```python
from build123d import *

# Parameters (mm, degrees)
SKETCH_1_W               = 31.1
SKETCH_1_H               = 31.1
SKETCH_1_W_2             = 21.1
SKETCH_1_H_2             = 21.1
EXTRUDE_1_DEPTH          = 60
SKETCH_2_R               = 1.55
CUT_EXTRUDE_1_DEPTH      = 73.445979875
CUT_EXTRUDE_2_DEPTH      = 71.444446197
CUT_EXTRUDE_2_DEPTH_BACK = 71.444446197
SKETCH_3_W               = 2.7
SKETCH_3_H               = 6
SKETCH_4_R               = 1.55
CUT_EXTRUDE_3_DEPTH      = 73.445979875
CUT_EXTRUDE_4_DEPTH      = 71.444446197
CUT_EXTRUDE_4_DEPTH_BACK = 71.444446197
SKETCH_5_W               = 3.5
SKETCH_5_H               = 6.2
FILLET_1_R               = 1.5
SKETCH_6_W               = 20.2
SKETCH_6_H               = 20.2
CUT_EXTRUDE_5_DEPTH      = 73.445979875
SKETCH_7_R               = 1.55
EXTRUDE_2_DEPTH          = 2.25
EXTRUDE_START            = 2.25
SKETCH_8_R               = 1.55
EXTRUDE_3_DEPTH          = 2.25


with BuildPart() as part:
    # 草图1 → 凸台-拉伸1 (new body)
    with BuildSketch(Plane(origin=(0, 0, 0), x_dir=(1, 0, 0), z_dir=(0, 1, 0))):
        with Locations((10.55, 10.55)):
            Rectangle(SKETCH_1_W, SKETCH_1_H)
        with Locations((10.55, 10.55)):
            Rectangle(SKETCH_1_W_2, SKETCH_1_H_2, mode=Mode.SUBTRACT)
    extrude(amount=EXTRUDE_1_DEPTH)

    # 草图2 → 切除-拉伸1 (cut, through all)
    with BuildSketch(Plane.ZY.offset(5)):
        with Locations((-23.6, 57)):
            Circle(SKETCH_2_R)
        with Locations((-23.6, 3)):
            Circle(SKETCH_2_R)
        with Locations((2.5, 3)):
            Circle(SKETCH_2_R)
        with Locations((2.5, 57)):
            Circle(SKETCH_2_R)
    extrude(amount=-CUT_EXTRUDE_1_DEPTH, mode=Mode.SUBTRACT)

    # 草图3 → 切除-拉伸2 (cut, two sides: drawn at the far end of the back side and taken through both)
    with BuildSketch(Plane.XY.offset(-21.1).offset(-CUT_EXTRUDE_2_DEPTH_BACK)):
        with Locations((6.2, 57)):
            Rectangle(SKETCH_3_W, SKETCH_3_H)
        with Locations((14.9, 57)):
            Rectangle(SKETCH_3_W, SKETCH_3_H)
        with Locations((14.9, 3)):
            Rectangle(SKETCH_3_W, SKETCH_3_H)
        with Locations((6.2, 3)):
            Rectangle(SKETCH_3_W, SKETCH_3_H)
    extrude(amount=CUT_EXTRUDE_2_DEPTH + CUT_EXTRUDE_2_DEPTH_BACK, mode=Mode.SUBTRACT)

    # 草图4 → 切除-拉伸3 (cut, through all)
    with BuildSketch(Plane(origin=(0, 0, -26.1), x_dir=(-1, 0, 0), z_dir=(0, 0, -1))):
        with Locations((-23.6, 53)):
            Circle(SKETCH_4_R)
        with Locations((2.5, 53)):
            Circle(SKETCH_4_R)
        with Locations((2.5, 7)):
            Circle(SKETCH_4_R)
        with Locations((-23.6, 7)):
            Circle(SKETCH_4_R)
    extrude(amount=-CUT_EXTRUDE_3_DEPTH, mode=Mode.SUBTRACT)

    # 草图5 → 切除-拉伸4 (cut, two sides: drawn at the far end of the back side and taken through both)
    with BuildSketch(Plane.ZY.offset(-21.1).offset(-CUT_EXTRUDE_4_DEPTH_BACK)):
        with Locations((-15.3, 53)):
            Rectangle(SKETCH_5_W, SKETCH_5_H)
        with Locations((-5.8, 53)):
            Rectangle(SKETCH_5_W, SKETCH_5_H)
        with Locations((-5.8, 7)):
            Rectangle(SKETCH_5_W, SKETCH_5_H)
        with Locations((-15.3, 7)):
            Rectangle(SKETCH_5_W, SKETCH_5_H)
    extrude(amount=CUT_EXTRUDE_4_DEPTH + CUT_EXTRUDE_4_DEPTH_BACK, mode=Mode.SUBTRACT)

    # 圆角1
    fillet_1_edges = [part.edges().sort_by_distance(p)[0] for p in [
        (14.9, 6, 0),
        (14.9, 6, -26.1),
        (14.9, 6, 5),
        (14.9, 54, 0),
        (14.9, 54, -26.1),
        (14.9, 54, 5),
        (6.2, 54, 0),
        (6.2, 54, -26.1),
        (6.2, 54, 5),
        (21.1, 49.9, -15.3),
        (21.1, 56.1, -15.3),
        (21.1, 49.9, -5.8),
        (21.1, 56.1, -5.8),
        (21.1, 10.1, -5.8),
        (21.1, 3.9, -5.8),
        (21.1, 10.1, -15.3),
        (21.1, 3.9, -15.3),
        (0, 3.9, -15.3),
        (0, 10.1, -15.3),
        (26.1, 3.9, -15.3),
        (26.1, 10.1, -15.3),
        (-5, 3.9, -15.3),
        (-5, 10.1, -15.3),
        (0, 3.9, -5.8),
        (0, 10.1, -5.8),
        (26.1, 3.9, -5.8),
        (26.1, 10.1, -5.8),
        (-5, 3.9, -5.8),
        (-5, 10.1, -5.8),
        (0, 56.1, -5.8),
        (0, 49.9, -5.8),
        (26.1, 56.1, -5.8),
        (26.1, 49.9, -5.8),
        (-5, 49.9, -5.8),
        (-5, 56.1, -5.8),
        (0, 56.1, -15.3),
        (0, 49.9, -15.3),
        (26.1, 56.1, -15.3),
        (26.1, 49.9, -15.3),
        (-5, 49.9, -15.3),
        (-5, 56.1, -15.3),
        (6.2, 54, -21.1),
        (14.9, 54, -21.1),
        (14.9, 6, -21.1),
        (6.2, 6, -21.1),
        (6.2, 6, 0),
        (6.2, 6, -26.1),
        (6.2, 6, 5),
    ]]
    fillet(fillet_1_edges, radius=FILLET_1_R)

    # 草图6 → 切除-拉伸5 (cut, through all)
    with BuildSketch(Plane.XY.offset(5)):
        with Locations((10.55, 30)):
            Rectangle(SKETCH_6_W, SKETCH_6_H)
    extrude(amount=-CUT_EXTRUDE_5_DEPTH, mode=Mode.SUBTRACT)

    # 草图7 → 凸台-拉伸2 (add)
    with BuildSketch(Plane.XY.offset(5)):
        Polygon((13.55, 0), (13.55, 7.5), (16.25, 7.5), (16.25, 0), (26.1, 0), (26.1, 60), (16.25, 60), (16.25, 52.5), (13.55, 52.5), (13.55, 60), (7.55, 60), (7.55, 52.5), (4.85, 52.5), (4.85, 60), (-5, 60), (-5, 0), (4.85, 0), (4.85, 7.5), (7.55, 7.5), (7.55, 0), align=None)
        with Locations(Location((23.6, 7, 0), (0, 0, 180))):
            Circle(SKETCH_7_R, mode=Mode.SUBTRACT)
        with Locations(Location((23.6, 53, 0), (0, 0, 180))):
            Circle(SKETCH_7_R, mode=Mode.SUBTRACT)
        with Locations(Location((-2.5, 53, 0), (0, 0, 180))):
            Circle(SKETCH_7_R, mode=Mode.SUBTRACT)
        with Locations(Location((-2.5, 7, 0), (0, 0, 180))):
            Circle(SKETCH_7_R, mode=Mode.SUBTRACT)
    extrude(amount=EXTRUDE_2_DEPTH)

    # 草图8 → 凸台-拉伸3 (add)
    with BuildSketch(Plane(origin=(0, 0, -26.1), x_dir=(-1, 0, 0), z_dir=(0, 0, -1)).offset(EXTRUDE_START)):
        Polygon((-7.55, 7.5), (-4.85, 7.5), (-4.85, 0), (5, 0), (5, 60), (-4.85, 60), (-4.85, 52.5), (-7.55, 52.5), (-7.55, 60), (-13.55, 60), (-13.55, 52.5), (-16.25, 52.5), (-16.25, 60), (-26.1, 60), (-26.1, 0), (-16.25, 0), (-16.25, 7.5), (-13.55, 7.5), (-13.55, 0), (-7.55, 0), align=None)
        with Locations((-23.6, 7)):
            Circle(SKETCH_8_R, mode=Mode.SUBTRACT)
        with Locations((2.5, 7)):
            Circle(SKETCH_8_R, mode=Mode.SUBTRACT)
        with Locations((2.5, 53)):
            Circle(SKETCH_8_R, mode=Mode.SUBTRACT)
        with Locations((-23.6, 53)):
            Circle(SKETCH_8_R, mode=Mode.SUBTRACT)
    extrude(amount=-EXTRUDE_3_DEPTH)


solid = part.part
```
Verification items for the finished model (mm, model axes). A direction names the side the tool comes from. Round coordinates to 2 decimals unless told otherwise and drop trailing zeros. Write each loop counter-clockwise with the first axis right and the second up, starting at its lowest first coordinate (ties: lowest second). Pieces come first, ordered by that corner, then holes.
1. Section check B-B on x = 2. Enter the section's corners in (y, z), plus the area to 3 significant figures.
2. Draft check along Z on faces 4 (the flat face through (0.45, 30, 3)), 5 (the cylindrical face through (21.106, 1.487, 2.164)), 6 (the cylindrical face through (6.22, 53.55, 4.57)), 7 (the flat face through (11, 0, -25)). Enter one of: +Z half, -Z half, draft (parallel to the pull), parting line (faces both ways), or undercut.
3. Section check C-C on y = 34. Enter the section's corners in (x, z), plus the area to 3 significant figures.
4. Access from +Z, -Z, +X, -X, +Y, -Y to the whole of each face (thin tool, end or side, straight path). Record for faces 1 (the cylindrical face through (21.53, 49.45, -15.32)), 2 (the cylindrical face through (6.22, 6.45, -21.53)), 3 (the flat face through (15, 7.5, 6)).
5. Scan lines: L1, parallel to Y at x = 10.35, z = -23.6; L2, parallel to Y at x = -2.5, z = -8.8; L3, parallel to Y at x = 21.75, z = 2.5. Record each from-to range of solid material in increasing order.
6. Section check D-D on z = -23.6. State how many separate pieces and enclosed holes the cut face has, plus the area to 3 significant figures.
7. Gauge pin test, flat ends, axial feed: P1, Ø3, axis at y = 3, z = -23.6, coming from the -X side; P2, Ø0.6, axis at x = 6, z = 3, coming from the -Y side. Record the tip position at first contact, or that the pin passes through.
8. Section check A-A on z = -11. Enter the section's corners in (x, y).
Answer:
1. outline: (0, -28.35) - (60, -28.35) - (60, -21.1) - (40.1, -21.1) - (40.1, -26.1) - (19.9, -26.1) - (19.9, -21.1) - (0, -21.1) - close; (0, 0) - (19.9, 0) - (19.9, 5) - (40.1, 5) - (40.1, 0) - (60, 0) - (60, 7.25) - (0, 7.25) - close; hole circle Ø3.1 at (3, -23.6); hole circle Ø3.1 at (3, 2.5); hole circle Ø3.1 at (57, -23.6); hole circle Ø3.1 at (57, 2.5)
1. area: 638 mm2
2. face 4: undercut
2. face 5: undercut
2. face 6: +Z half
2. face 7: draft
3. outline: (-5, -28.35) - (26.1, -28.35) - (26.1, 7.25) - (-5, 7.25) - close; hole (0, -21.1) - (0.45, -21.1) - (0.45, -26.1) - (20.65, -26.1) - (20.65, -21.1) - (21.1, -21.1) - (21.1, 0) - (20.65, 0) - (20.65, 5) - (0.45, 5) - (0.45, 0) - (0, 0) - close
3. area: 460 mm2
4. face 1: none
4. face 2: -Y
4. face 3: +Z, -Y
5. L1: y = 0 to 1.45, 4.55 to 19.9, 40.1 to 55.45, 58.55 to 60
5. L2: y = 0 to 5.45, 8.55 to 51.45, 54.55 to 60
5. L3: y = 0 to 1.45, 4.55 to 55.45, 58.55 to 60
6. separate pieces: 7
6. enclosed holes: 5
6. area: 1,200 mm2
7. P1: passes through
7. P2: stops at y = 6
8. outline: (-5, 0) - (0, 0) - (0, 60) - (-5, 60) - close; (21.1, 0) - (26.1, 0) - (26.1, 60) - (21.1, 60) - close; hole circle Ø3.1 at (-2.5, 7); hole circle Ø3.1 at (-2.5, 53); hole circle Ø3.1 at (23.6, 7); hole circle Ø3.1 at (23.6, 53)
